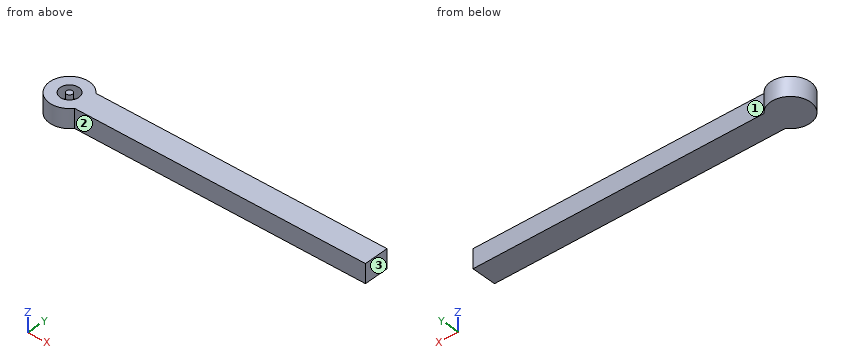
from build123d import *

# Parameters (mm, degrees)
SKETCH_1_R        = 3.05
EXTRUDE_1_DEPTH   = 4.2
SKETCH_1_R_2      = 1
EXTRUDE_1_2_DEPTH = 4.2
EXTRUDE_START     = -2
SKETCH_1_4_R      = 3.05
SKETCH_1_4_R_2    = 1
EXTRUDE_2_DEPTH   = 2


with BuildPart() as part:
    # Sketch 1 → Extrude 1 (new body)
    with BuildSketch(Plane.XY):
        with BuildLine():
            Line((5.123475383, 4), (100, 4))
            Line((100, 4), (100, -4))
            Line((100, -4), (5.123475383, -4))
            ThreePointArc((5.123475383, -4), (-6.5, 0), (5.123475383, 4))
        make_face()
        Circle(SKETCH_1_R, mode=Mode.SUBTRACT)
    extrude(amount=EXTRUDE_1_DEPTH)



with BuildPart() as body_2:
    # Sketch 1 → Extrude 1 2 (new body)
    with BuildSketch(Plane.XY):
        Circle(SKETCH_1_R_2)
    extrude(amount=EXTRUDE_1_2_DEPTH)


with BuildPart() as part_1:
    add(part.part)

    add(body_2.part)  # Extrude 2 merges body 2
    # Sketch 1_4 → Extrude 2 (add)
    # profile 1 of 3: a face of its own
    with BuildSketch(Plane.XY.offset(EXTRUDE_START)):
        with BuildLine():
            Line((5.123475383, 4), (100, 4))
            Line((100, 4), (100, -4))
            Line((100, -4), (5.123475383, -4))
            ThreePointArc((5.123475383, -4), (-6.5, 0), (5.123475383, 4))
        make_face()
        Circle(SKETCH_1_4_R, mode=Mode.SUBTRACT)
    # profile 2 of 3: a face of its own
    with BuildSketch(Plane.XY.offset(EXTRUDE_START)):
        Circle(SKETCH_1_4_R)
        Circle(SKETCH_1_4_R_2, mode=Mode.SUBTRACT)
    # profile 3 of 3: a face of its own
    with BuildSketch(Plane.XY.offset(EXTRUDE_START)):
        Circle(SKETCH_1_4_R_2)
    extrude(amount=EXTRUDE_2_DEPTH)


solid = part_1.part
Model file for the job. Use its own axes, mm. Face numbers are marked on the shaded views. A direction names the side the tool comes from. Give positions to 0.01 mm unless a question says otherwise; leave off trailing zeros. Loops run counter-clockwise (first coordinate to the right, second up) from the corner with the lowest first, then second, coordinate; pieces in that order, holes last.
1) Tool access for the marked faces 1, 2 and 3: list every direction of +Z, -Z, +X, -X, +Y, -Y with a clear straight run to the whole face (end or side of a thin tool).
2) Saw through at B-B (y = 0). Write the cut outline in (x, z), plus the area to 3 significant figures.
3) Wall check: line 1 (Y direction, x = 0, z = 2.8); line 2 (Y direction, x = 71.5, z = -0.5); line 3 (X direction, y = -1.25, z = 0.75). Give the ranges that are in metal, low to high.
4) Saw through at C-C (x = 0). Write the cut outline in (y, z).
5) Saw through at A-A (z = 1.75). Write the cut outline in (x, y), plus the area to 3 significant figures.
6) Saw through at D-D (x = 63). Write the cut outline in (y, z), plus the area to 3 significant figures.
7) Flat gauge pins, fed straight in: pin 1 Ø1 at (x, z) = (27, 0.5) entering from +Y; pin 2 Ø3 at (x, z) = (67, 0.5) entering from -Y; pin 3 Ø2 at (y, z) = (-2, 0) entering from -X. Where does each tip first touch, or does it go through?
Answer block:
1. face 1: +Z, -Z, +X, +Y
1. face 2: +Z, -Z, +X, -Y
1. face 3: +Z, -Z, +X, +Y, -Y
2. outline: (-6.5, -2) - (100, -2) - (100, 4.2) - (3.05, 4.2) - (3.05, 0) - (1, 0) - (1, 4.2) - (-1, 4.2) - (-1, 0) - (-3.05, 0) - (-3.05, 4.2) - (-6.5, 4.2) - close
2. area: 643 mm2
3. line 1: y = -6.5 to -3.05, -1 to 1, 3.05 to 6.5
3. line 2: y = -4 to 4
3. line 3: x = -6.38 to -2.78, 2.78 to 100
4. outline: (-6.5, -2) - (6.5, -2) - (6.5, 4.2) - (3.05, 4.2) - (3.05, 0) - (1, 0) - (1, 4.2) - (-1, 4.2) - (-1, 0) - (-3.05, 0) - (-3.05, 4.2) - (-6.5, 4.2) - close
5. outline: circle Ø2 at (0, 0); (5.12, -4) - (100, -4) - (100, 4) - (5.12, 4) arc R6.5 ccw (long way) to start; hole circle Ø6.1 at (0, 0)
5. area: 858 mm2
6. outline: (-4, -2) - (4, -2) - (4, 4.2) - (-4, 4.2) - close
6. area: 49.6 mm2
7. pin 1: stops at y = 4
7. pin 2: stops at y = -4
7. pin 3: stops at x = -6.42
